Part model, mm, in its own coordinate system. A direction names the side the tool comes from. Give positions to 0.01 mm unless a question says otherwise; leave off trailing zeros. Order: outer loops, then holes, each group sorted by start corner. A loop starts at its lowest first (then second) coordinate and runs counter-clockwise, first axis right, second up. Notation, with made-up numbers: (-40, 41) - (-22, 41) arc R24 cw to (-22, 55) - close; hole circle Ø11 at (53.25, 60). An arc over 180 degrees is marked (long way). Use one line per item in the form item = value. Start each with the question number.
1. Band-saw the part on B-B, the plane x = 0. List the corners of the cut face in (y, z), plus the area to 3 significant figures.
2. Band-saw the part on D-D, the plane x = 19.5. List the corners of the cut face in (y, z), plus the area to 3 significant figures.
3. Drill centre lines: line 1 (X direction, y = 47, z = 2.4); line 2 (Y direction, x = -16, z = 4.5); line 3 (Y direction, x = 34, z = 1.1). Where is each one in solid material? Low to high.
4. Pull direction X, two halves, no side cores. Call faces 3 (the face through (-26, 53, 5)), 4 (the face through (32.267, 68.208, 2.465)), 5 (the face through (-58.37, 31.5, 2.46)), 6 (the face through (35.64, 4.66, 2.46)): +X half, -X half, draft (parallel to the pull), parting line (faces both ways), or undercut.
5. Band-saw the part on C-C, the plane y = 58.5. List the corners of the cut face in (x, z).
6. Pin check, flat tips, straight feed: P1, Ø1.5, axis at y = 23.5, z = 1.5, coming from the -X side; P2, Ø19, axis at x = -32.5, y = 40, coming from the -Z side; P3, Ø1.5, axis at y = 56.5, z = 1.5, coming from the -X side; P4, Ø4, axis at x = 37, y = 54.5, coming from the -Z side. Stop position of each tip, or through.
7. Tool access for faces 1 (the face through (0, 89, 2)), 2 (the face through (-35.125, 4.102, 2.465)): list every direction of +Z, -Z, +X, -X, +Y, -Y with a clear straight run to the whole face (end or side of a thin tool).
8. Band-saw the part on A-A, the plane z = 3.55. List the corners of the cut face in (x, y), plus the area to 3 significant figures.
from build123d import *

# Parameters (mm, degrees)
SKETCH2_R           = 10.5
BOSS_EXTRUDE1_DEPTH = 5


with BuildPart() as part:
    # Sketch2 → Boss-Extrude1 (new body)
    with BuildSketch(Plane.XY):
        with BuildLine():
            Line((53.88428711, 24.382034423), (16.88428711, -15.617965577))
            ThreePointArc((16.88428711, -15.617965577), (0, -23), (-16.88428711, -15.617965577))
            Line((-16.88428711, -15.617965577), (-53.88428711, 24.382034423))
            ThreePointArc((-53.88428711, 24.382034423), (-58.416566059, 31.613660022), (-60, 40))
            ThreePointArc((-60, 40), (0, 100), (60, 40))
            ThreePointArc((60, 40), (58.416566059, 31.613660022), (53.88428711, 24.382034423))
        make_face()
        with Locations((32.5, 40)):
            Circle(SKETCH2_R, mode=Mode.SUBTRACT)
        with Locations(Location((-32.5, 40, 0), (0, 0, 180))):
            Circle(SKETCH2_R, mode=Mode.SUBTRACT)
        with BuildLine():
            Line((8.809193275, -8.148503779), (23.364034903, 7.586460143))
            ThreePointArc((23.364034903, 7.586460143), (27.338026386, 18.431860253), (22.426271655, 28.886044933))
            ThreePointArc((22.426271655, 28.886044933), (17.542994151, 41.134890312), (24.218531469, 52.506689369))
            ThreePointArc((24.218531469, 52.506689369), (32.255432897, 68.469423949), (22.572828784, 83.491003675))
            ThreePointArc((22.572828784, 83.491003675), (0, 89), (-22.572828784, 83.491003675))
            ThreePointArc((-22.572828784, 83.491003675), (-32.255432897, 68.469423949), (-24.218531469, 52.506689369))
            ThreePointArc((-24.218531469, 52.506689369), (-17.542994151, 41.134890312), (-22.426271655, 28.886044933))
            ThreePointArc((-22.426271655, 28.886044933), (-27.338026386, 18.431860253), (-23.364034903, 7.586460143))
            Line((-23.364034903, 7.586460143), (-8.809193275, -8.148503779))
            ThreePointArc((-8.809193275, -8.148503779), (0, -12), (8.809193275, -8.148503779))
        make_face(mode=Mode.SUBTRACT)
    extrude(amount=BOSS_EXTRUDE1_DEPTH)


solid = part.part
From the geometry:
q1.outline = (-23, 0) - (-12, 0) - (-12, 5) - (-23, 5) - close; (89, 0) - (100, 0) - (100, 5) - (89, 5) - close
q1.area = 110 mm²
q2.outline = (-12.79, 0) - (3.41, 0) - (3.41, 5) - (-12.79, 5) - close; (32.52, 0) - (47.48, 0) - (47.48, 5) - (32.52, 5) - close; (84.95, 0) - (96.74, 0) - (96.74, 5) - (84.95, 5) - close
q2.area = 215 mm²
q3.line_1 = -59.59 to -40.33, -24.67 to -19.23, 19.23 to 24.67, 40.33 to 59.59
q3.line_2 = -16.52 to -0.37, 86.31 to 97.83
q3.line_3 = 2.89 to 29.61, 50.39 to 89.44
q4.face_3 = draft
q4.face_4 = undercut
q4.face_5 = -X half
q4.face_6 = +X half
q5.outline = (-57.08, 0) - (-29.86, 0) - (-29.86, 5) - (-57.08, 5) - close; (29.86, 0) - (57.08, 0) - (57.08, 5) - (29.86, 5) - close
q6.P1 = -53.76
q6.P2 = through
q6.P3 = -57.9
q6.P4 = 0
q7.face_1 = +Z, -Z
q7.face_2 = +Z, -Z, -X, -Y
q8.outline = (-60, 40) arc R23 ccw to (-53.88, 24.38) - (-16.88, -15.62) arc R23 ccw to (16.88, -15.62) - (53.88, 24.38) arc R23 ccw to (60, 40) arc R60 ccw to start; hole circle Ø21 at (-32.5, 40); hole (-24.22, 52.51) arc R15 cw to (-22.43, 28.89) arc R15 ccw to (-23.36, 7.59) - (-8.81, -8.15) arc R12 ccw to (8.81, -8.15) - (23.36, 7.59) arc R15 ccw to (22.43, 28.89) arc R15 cw to (24.22, 52.51) arc R18 ccw to (22.57, 83.49) arc R49 ccw to (-22.57, 83.49) arc R18 ccw to start; hole circle Ø21 at (32.5, 40)
q8.area = 5,200 mm²
